```python
from build123d import *

# Parameters (mm, degrees)
CROQUIS1_W              = 28
CROQUIS1_H              = 30
SALIENTE_EXTRUIR1_DEPTH = 30
CROQUIS2_W              = 22
CROQUIS2_H              = 24
CORTAR_EXTRUIR1_DEPTH   = 25
CORTAR_EXTRUIR3_START   = -30
CORTAR_EXTRUIR3_DEPTH   = 30
CROQUIS3_R              = 2
CORTAR_EXTRUIR4_DEPTH   = 5
CORTAR_EXTRUIR5_START   = -30
CROQUIS6_R              = 1.5
CORTAR_EXTRUIR5_DEPTH   = 30
CROQUIS8_W              = 30
CROQUIS8_H              = 78
SALIENTE_EXTRUIR2_DEPTH = 2
CROQUIS9_W              = 3.3
CROQUIS9_H              = 3
SALIENTE_EXTRUIR3_DEPTH = 48
CROQUIS10_W             = 30
CROQUIS10_H             = 2
SALIENTE_EXTRUIR4_DEPTH = 5.3
CROQUIS11_W             = 24
CROQUIS11_H             = 48
CORTAR_EXTRUIR6_DEPTH   = 1
SALIENTE_EXTRUIR5_DEPTH = 3
REDONDEO2_R             = 2


with BuildPart() as part:
    # Croquis1 → Saliente-Extruir1 (new body)
    with BuildSketch(Plane.XY):
        with Locations((-25.946619217, -0.658362989)):
            Rectangle(CROQUIS1_W, CROQUIS1_H)
    extrude(amount=SALIENTE_EXTRUIR1_DEPTH)

    # Croquis2 → Cortar-Extruir1 (cut)
    with BuildSketch(Plane.XZ.offset(15.658362989)):
        with Locations((-25.946619217, 15)):
            Rectangle(CROQUIS2_W, CROQUIS2_H)
    extrude(amount=-CORTAR_EXTRUIR1_DEPTH, mode=Mode.SUBTRACT)

    # Croquis5 → Cortar-Extruir3 (cut)
    with BuildSketch(Plane.XY.offset(30).offset(CORTAR_EXTRUIR3_START)):
        with BuildLine():
            Line((-18.463304444, 14.341637011), (-33.429933991, 14.341637011))
            ThreePointArc((-33.429933991, 14.341637011), (-25.946619217, 10.341637011), (-18.463304444, 14.341637011))
        make_face()
    extrude(amount=CORTAR_EXTRUIR3_DEPTH, mode=Mode.SUBTRACT)

    # Croquis3 → Cortar-Extruir4 (cut)
    with BuildSketch(Plane.XZ.offset(-9.341637011)):
        with Locations((-25.946619217, 15)):
            Circle(CROQUIS3_R)
    extrude(amount=-CORTAR_EXTRUIR4_DEPTH, mode=Mode.SUBTRACT)

    # Croquis6 → Cortar-Extruir5 (cut)
    with BuildSketch(Plane.XY.offset(30).offset(CORTAR_EXTRUIR5_START)):
        with Locations((-27.946619217, -2.658362989)):
            Circle(CROQUIS6_R)
    extrude(amount=CORTAR_EXTRUIR5_DEPTH, mode=Mode.SUBTRACT)

    # Croquis8 → Saliente-Extruir2 (add)
    with BuildSketch(Plane(origin=(-11.946619217, 0, 0), x_dir=(0, 0, -1), z_dir=(1, 0, 0))):
        with Locations((-15, -24.658362989)):
            Rectangle(CROQUIS8_W, CROQUIS8_H)
    extrude(amount=SALIENTE_EXTRUIR2_DEPTH)

    # Croquis9 → Saliente-Extruir3 (add)
    with BuildSketch(Plane.XZ.offset(15.658362989)):
        with Locations((-13.596619217, 1.5)):
            Rectangle(CROQUIS9_W, CROQUIS9_H)
        with Locations((-13.596619217, 28.5)):
            Rectangle(CROQUIS9_W, CROQUIS9_H)
    extrude(amount=SALIENTE_EXTRUIR3_DEPTH)

    # Croquis10 → Saliente-Extruir4 (add)
    with BuildSketch(Plane(origin=(-9.946619217, 0, 0), x_dir=(0, 0, -1), z_dir=(1, 0, 0))):
        with Locations((-15, -64.658362989)):
            Rectangle(CROQUIS10_W, CROQUIS10_H)
    extrude(amount=-SALIENTE_EXTRUIR4_DEPTH)

    # Croquis11 → Cortar-Extruir6 (cut)
    with BuildSketch(Plane.ZY.offset(11.946619217)):
        with Locations((15, -39.658362989)):
            Rectangle(CROQUIS11_W, CROQUIS11_H)
    extrude(amount=-CORTAR_EXTRUIR6_DEPTH, mode=Mode.SUBTRACT)

    # Croquis12 → Saliente-Extruir5 (add)
    with BuildSketch(Plane.XY.offset(30)):
        with BuildLine():
            Line((-15.246619217, -15.658362989), (-15.246619217, -24.658362989))
            Line((-15.246619217, -24.658362989), (-15.246619217, -25.658362989))
            add(Edge.make_bspline(
                [(-15.246619217, -25.658362989), (-15.454297932, -24.784354335), (-16.276669262, -23.769291156), (-17.060396799, -21.819515511), (-25.742756364, -19.637986616), (-31.719204445, -16.94099226), (-39.946619217, -17.158362989)],
                knots=[0, 0, 0, 0, 0.094483023, 0.145649735, 0.216240506, 1, 1, 1, 1], degree=3))
            Line((-39.946619217, -17.158362989), (-39.946619217, -15.658362989))
            Line((-39.946619217, -15.658362989), (-15.246619217, -15.658362989))
        make_face()
    saliente_extruir5 = extrude(amount=-SALIENTE_EXTRUIR5_DEPTH)

    # Simetría2: Saliente-Extruir5 across plane
    add(saliente_extruir5.mirror(Plane(origin=(0, 0, 15), x_dir=(1, 0, 0), z_dir=(0, 0, -1))))

    # Redondeo2
    redondeo2_edges = [part.edges().sort_by_distance(p)[0] for p in [
        (-14.20496183, 14.341637011, 30),
        (-36.688276604, 14.341637011, 0),
        (-36.688276604, 14.341637011, 30),
        (-39.946619217, -1.408362989, 30),
        (-14.20496183, 14.341637011, 0),
        (-9.946619217, -25.658362989, 30),
        (-9.946619217, -25.658362989, 0),
        (-9.946619217, 14.341637011, 15),
        (-39.946619217, -1.408362989, 0),
        (-39.946619217, 14.341637011, 15),
        (-9.946619217, -65.658362989, 15),
    ]]
    fillet(redondeo2_edges, radius=REDONDEO2_R)


solid = part.part
```
The model under review builds one solid part; all positions refer to its coordinate system, in mm. A direction names the side the tool comes from. Coordinates: 2 decimals unless noted, no trailing zeros. Write each loop counter-clockwise with the first axis right and the second up, starting at its lowest first coordinate (ties: lowest second). Pieces come first, ordered by that corner, then holes. Notation, with made-up numbers: (31, -4.5) - (68, -4.5) arc R19 cw to (68, 16.5) - close; hole circle Ø7 at (-40, 14). An arc over 180 degrees is marked (long way). Answer in a Markdown table with one row per item. Add a question column.
Q1. Consider section A-A on z = 15. Give the boundary of the cut face in (x, y).
Q2. Consider section B-B on y = -45. Give the boundary of the cut face in (x, z), then the cut area to 3 significant figures.
Q3. Clearance check with flat-ended pins moving along their axes: pin 1 (3 mm diameter, centred on x = -25.5, z = 5, fed in from -Y); pin 2 (7 mm diameter, centred on y = -35, z = 20, fed in from -X); pin 3 (10 mm diameter, centred on x = -30.5, z = 5.5, fed in from -Y). State where each tip first meets the part, or that it passes through.
Q4. To check wall thickness, follow line 1 along X through (y, z) = (4, 12.5); line 2 along X through (y, z) = (10, 15); line 3 along X through (y, z) = (-61.5, 6.5). State the ranges of each line that lie inside material, in increasing order. Write a range as from..to.
Q5. Draft analysis for pull direction Z (two halves, no side actions). For faces 4 (the face through (-39.345, -2.615, 0.57)), 5 (the face through (-9.947, -25, 15)), 6 (the face through (-22, -10, 3)), 7 (the face through (-29, 9.342, 15)), state which applies: +Z half, -Z half, draft (parallel to the pull), parting line (faces both ways), or undercut.
Q6. For faces 1 (the face through (-39.947, -3, 15)), 2 (the face through (-10.947, -39, 15)), 3 (the face through (-14.947, -3, 15)), list the 3-axis set-ups (+Z, -Z, +X, -X, +Y, -Y) from which the entire face can be reached by the end or side of a thin tool; tool diameter is ignored.
Answers below:
| question | item | result |
|---|---|---|
| 1 | outline | (-39.95, -15.66) - (-36.95, -15.66) - (-36.95, 9.34) - (-27.95, 9.34) - (-27.95, 10.57) arc R9 cw to (-33.43, 14.34) - (-37.95, 14.34) arc R2 ccw to (-39.95, 12.34) - close; (-23.95, 9.34) - (-14.95, 9.34) - (-14.95, -15.66) - (-10.95, -15.66) - (-10.95, -63.66) - (-15.25, -63.66) - (-15.25, -65.66) - (-11.95, -65.66) arc R2 ccw to (-9.95, -63.66) - (-9.95, 12.34) arc R2 ccw to (-11.95, 14.34) - (-18.46, 14.34) arc R9 cw to (-23.95, 10.57) - close |
| 2 | outline | (-15.25, 0) - (-11.95, 0) arc R2 ccw to (-9.95, 2) - (-9.95, 28) arc R2 ccw to (-11.95, 30) - (-15.25, 30) - (-15.25, 27) - (-10.95, 27) - (-10.95, 3) - (-15.25, 3) - close |
| 2 | area | 54.1 mm² |
| 3 | pin 1 | y = 9.34 |
| 3 | pin 2 | x = -10.95 |
| 3 | pin 3 | y = -19.24 |
| 4 | line 1 | -39.95..-36.95, -14.95..-9.95 |
| 4 | line 2 | -39.95..-27.95, -23.95..-9.95 |
| 4 | line 3 | -10.95..-9.95 |
| 5 | face 4 | -Z half |
| 5 | face 5 | draft |
| 5 | face 6 | undercut |
| 5 | face 7 | undercut |
| 6 | face 1 | +Z, -Z, -X, +Y, -Y |
| 6 | face 2 | -X |
| 6 | face 3 | none |
